Geometry: final body of the model. Coordinates: model frame, mm. Face numbers are marked on the shaded views. A direction names the side the tool comes from. Round coordinates to 2 decimals unless told otherwise and drop trailing zeros. Loops run counter-clockwise (first coordinate to the right, second up) from the corner with the lowest first, then second, coordinate; pieces in that order, holes last. Notation, with made-up numbers: (34.25, 80) - (67.25, 80) arc R17 ccw to (67.25, 110) - close; hole circle Ø8 at (-20, 74). An arc over 180 degrees is marked (long way). Return JSON: item names as keys, results as strings. Group by question number.
1. Draft query along X for the marked faces 1, 2, 3 and 4. Return one class per face: +X half, -X half, draft (parallel to the pull), parting line (faces both ways), or undercut.
2. Section D-D on x = 12. Return loops of the section in (y, z), and give its area (3 significant figures).
3. First-contact query: pin 1 Ø6 at (x, z) = (2, 22) entering from -Y; pin 2 Ø6.5 at (x, y) = (42, -6.5) entering from +Z; pin 3 Ø10 at (x, z) = (17.5, 29.5) entering from -Y; pin 4 Ø2.5 at (y, z) = (3.5, 9.5) entering from -X. Flat tips, straight axial feed; report the tip coordinate or a pass-through.
4. Section C-C on y = -3.5. Return loops of the section in (x, z).
5. Section A-A on x = 38.5. Return loops of the section in (y, z).
6. Material intervals for probe 1 along X at (y, z) = (-9, 19.5); probe 2 along Z at (x, y) = (43, -3); probe 3 along Z at (x, y) = (-22, -8), sorted ascending.
7. Section B-B on y = -27.5. Return loops of the section in (x, z).
8. Set-up query: the marked faces 5, 6 and 7. Return all of +Z, -Z, +X, -X, +Y, -Y with unobstructed straight access to the full face (end or side cutting, diameter ignored); none if empty.
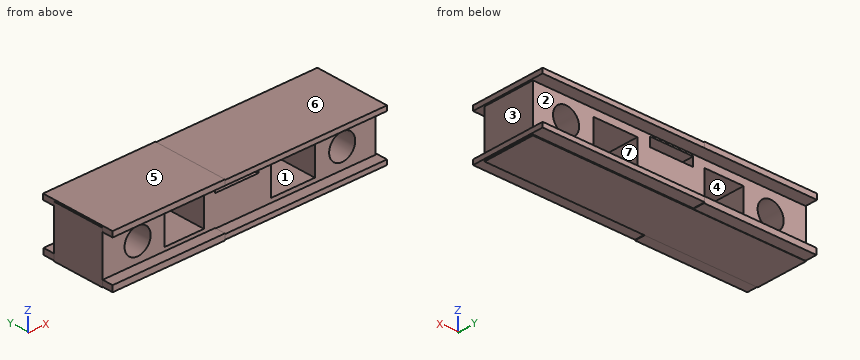
from build123d import *

# Parameters (mm, degrees)
F0_W     = 132.736026
F0_H     = 24.608365
F0_W_2   = 19.050001
F0_H_2   = 14.360769
F0_W_3   = 21.394616
F0_R     = 6.3373
F1_DEPTH = 25.4
F2_W     = 36.634613
F2_H     = 2.344616
F3_DEPTH = 78.74
F4_W     = 36.634616
F4_H     = 2.637692
F4_W_2   = 36.341539
F4_H_2   = 2.930769
F5_DEPTH = 54.61
F6_W     = 21.052692
F6_H     = 4.396153
F7_DEPTH = 50.8


with BuildPart() as f1:
    # F0 (on Front) → F1 (new body)
    with BuildSketch(Plane.XZ):
        with Locations((11.576537, 19.929231)):
            Rectangle(F0_W, F0_H)
        with Locations((-14.946923, 19.636154)):
            Rectangle(F0_W_2, F0_H_2, mode=Mode.SUBTRACT)
        with Locations((37.806922, 19.636154)):
            Rectangle(F0_W_3, F0_H_2, mode=Mode.SUBTRACT)
        with Locations((-37.640192, 20.053516)):
            Circle(F0_R, mode=Mode.SUBTRACT)
        with Locations((61.787547, 20.053516)):
            Circle(F0_R, mode=Mode.SUBTRACT)
    extrude(amount=F1_DEPTH)

    # F2 (on Right) → F3 (join)
    with BuildSketch(Plane.YZ):
        with Locations((-12.30923, 31.505771)):
            Rectangle(F2_W, F2_H)
        with Locations((-12.30923, 9.231923)):
            Rectangle(F2_W, F2_H)
    extrude(amount=F3_DEPTH)

    # F4 (on Right) → F5 (join)
    with BuildSketch(Plane.YZ):
        with Locations((-12.309231, 31.652309)):
            Rectangle(F4_W, F4_H)
        with Locations((-12.455769, 9.231924)):
            Rectangle(F4_W_2, F4_H_2)
    extrude(amount=-F5_DEPTH)

    # F6 (on Front) → F7 (cut)
    with BuildSketch(Plane.XZ):
        with Locations((10.526346, 27.256155)):
            Rectangle(F6_W, F6_H)
    extrude(amount=F7_DEPTH, mode=Mode.SUBTRACT)


solid = f1.part
Taken from the geometry:
{
 "1": {"face 1": "undercut", "face 2": "draft", "face 3": "+X half", "face 4": "undercut"},
 "2": {"outline": "(-30.63, 8.06) - (-25.4, 8.06) - (-25.4, 7.63) - (0, 7.63) - (0, 8.06) - (6.01, 8.06) - (6.01, 10.4) - (0, 10.4) - (0, 25.06) - (-25.4, 25.06) - (-25.4, 10.4) - (-30.63, 10.4) - close; (-30.63, 30.33) - (-25.4, 30.33) - (-25.4, 29.45) - (0, 29.45) - (0, 30.33) - (6.01, 30.33) - (6.01, 32.68) - (-30.63, 32.68) - close", "area": "577 mm2"},
 "3": {"pin 1": "y = -25.4", "pin 2": "z = 32.68", "pin 3": "y = -30.63", "pin 4": "x = -54.61"},
 "4": {"outline": "(-54.79, 7.63) - (77.94, 7.63) - (77.94, 8.06) - (78.74, 8.06) - (78.74, 10.4) - (77.94, 10.4) - (77.94, 30.33) - (78.74, 30.33) - (78.74, 32.68) - (0, 32.68) - (0, 32.97) - (-54.61, 32.97) - (-54.61, 32.23) - (-54.79, 32.23) - close; hole circle Ø12.67 at (-37.64, 20.05); hole (-24.47, 12.46) - (-5.42, 12.46) - (-5.42, 26.82) - (-24.47, 26.82) - close; hole (0, 25.06) - (21.05, 25.06) - (21.05, 29.45) - (0, 29.45) - close; hole (27.11, 12.46) - (48.5, 12.46) - (48.5, 26.82) - (27.11, 26.82) - close; hole circle Ø12.67 at (61.79, 20.05)"},
 "5": {"outline": "(-30.63, 8.06) - (-25.4, 8.06) - (-25.4, 7.63) - (0, 7.63) - (0, 8.06) - (6.01, 8.06) - (6.01, 10.4) - (0, 10.4) - (0, 12.46) - (-25.4, 12.46) - (-25.4, 10.4) - (-30.63, 10.4) - close; (-30.63, 30.33) - (-25.4, 30.33) - (-25.4, 26.82) - (0, 26.82) - (0, 30.33) - (6.01, 30.33) - (6.01, 32.68) - (-30.63, 32.68) - close"},
 "6": {"probe 1": "-54.79 to -43.95, -31.33 to -24.47, -5.42 to 27.11, 48.5 to 55.47, 68.1 to 77.94", "probe 2": "7.63 to 12.46, 26.82 to 32.68", "probe 3": "7.63 to 12.46, 26.82 to 32.97"},
 "7": {"outline": "(-54.61, 7.77) - (0, 7.77) - (0, 8.06) - (78.74, 8.06) - (78.74, 10.4) - (0, 10.4) - (0, 10.7) - (-54.61, 10.7) - close; (-54.61, 30.33) - (78.74, 30.33) - (78.74, 32.68) - (0, 32.68) - (0, 32.97) - (-54.61, 32.97) - close"},
 "8": {"face 5": "+Z, +X, -X, +Y, -Y", "face 6": "+Z, +X, +Y, -Y", "face 7": "+Y, -Y"}
}
